Design review of the part built by this model. Coordinates are the model's own, in mm. A direction names the side the tool comes from. Coordinates: 2 decimals unless noted, no trailing zeros. Order: outer loops, then holes, each group sorted by start corner. A loop starts at its lowest first (then second) coordinate and runs counter-clockwise, first axis right, second up. Notation, with made-up numbers: (4.5, 70) -> (25.5, 70) arc R30 ccw to (25.5, 109) -> close; hole circle Ø1 at (10.5, 38). An arc over 180 degrees is marked (long way). Write item = value, one per line.
```python
from build123d import *

# Parameters (mm, degrees)
SKETCH_1_W      = 50
SKETCH_1_H      = 70
SKETCH_1_R      = 2.15
SKETCH_1_W_2    = 3.5
SKETCH_1_H_2    = 45
EXTRUDE_1_DEPTH = 5
FILLET_1_R      = 2
FILLET_2_R      = 2


with BuildPart() as part:
    # 草圖1 → 填料-伸長1 (new body)
    with BuildSketch(Plane(origin=(0, 0, 0), x_dir=(1, 0, 0), z_dir=(0, 1, 0))):
        Rectangle(SKETCH_1_W, SKETCH_1_H)
        with Locations(Location((-15.5, 25, 0), (0, 0, 270))):
            Circle(SKETCH_1_R, mode=Mode.SUBTRACT)
        with Locations(Location((15.5, 25, 0), (0, 0, 270))):
            Circle(SKETCH_1_R, mode=Mode.SUBTRACT)
        with Locations((-15.1, -7.5)):
            Rectangle(SKETCH_1_W_2, SKETCH_1_H_2, mode=Mode.SUBTRACT)
        with Locations((15.1, -7.5)):
            Rectangle(SKETCH_1_W_2, SKETCH_1_H_2, mode=Mode.SUBTRACT)
    extrude(amount=EXTRUDE_1_DEPTH)

    # 圓角1
    # the kernel refuses this fillet: 2 mm, written as the material it adds along each edge
    with BuildSketch(Plane(origin=(16.85, 0, 30), x_dir=(0, 0, -1), z_dir=(0, 1, 0)), Plane(origin=(-13.35, 0, 30), x_dir=(0, 0, -1), z_dir=(0, 1, 0))) as fillet_1_piece_1:
        with BuildLine():
            CenterArc((FILLET_1_R, FILLET_1_R), FILLET_1_R, 180, 90)
            Line((0, FILLET_1_R), (0, 0))
            Line((0, 0), (FILLET_1_R, 0))
        make_face()
    extrude(amount=5)
    with BuildSketch(Plane(origin=(13.35, 0, 30), x_dir=(0, 0, -1), z_dir=(0, 1, 0)), Plane(origin=(-16.85, 0, 30), x_dir=(0, 0, -1), z_dir=(0, 1, 0)), Plane(origin=(16.85, 0, -15), x_dir=(0, 0, 1), z_dir=(0, 1, 0)), Plane(origin=(13.35, 0, -15), x_dir=(1, 0, 0), z_dir=(0, 1, 0)), Plane(origin=(-13.35, 0, -15), x_dir=(0, 0, 1), z_dir=(0, 1, 0)), Plane(origin=(-16.85, 0, -15), x_dir=(1, 0, 0), z_dir=(0, 1, 0))) as fillet_1_piece_2:
        with BuildLine():
            CenterArc((FILLET_1_R, -FILLET_1_R), FILLET_1_R, 90, 90)
            Line((0, -FILLET_1_R), (0, 0))
            Line((0, 0), (FILLET_1_R, 0))
        make_face()
    extrude(amount=5)

    # 圓角2
    fillet_2_edges = [part.edges().sort_by_distance(p)[0] for p in [
        (25, 2.5, 35),
        (-25, 2.5, 35),
        (-25, 2.5, -35),
        (25, 2.5, -35),
    ]]
    fillet(fillet_2_edges, radius=FILLET_2_R)


solid = part.part
```
(1) We need section C-C (z = -25). Write out the cut boundary in (x, y).
Report:
outline = (-25, 0) -> (-17.65, 0) -> (-17.65, 5) -> (-25, 5) -> close; (-13.35, 0) -> (13.35, 0) -> (13.35, 5) -> (-13.35, 5) -> close; (17.65, 0) -> (25, 0) -> (25, 5) -> (17.65, 5) -> close
(2) We need section B-B (z = 8). Write out the cut boundary in (x, y), and give its area (3 significant figures).
Report:
outline = (-25, 0) -> (-16.85, 0) -> (-16.85, 5) -> (-25, 5) -> close; (-13.35, 0) -> (13.35, 0) -> (13.35, 5) -> (-13.35, 5) -> close; (16.85, 0) -> (25, 0) -> (25, 5) -> (16.85, 5) -> close
area = 215 mm²
(3) We need section A-A (y = 3.3). Write out the cut boundary in (x, z).
Report:
outline = (-25, -33) arc R2 ccw to (-23, -35) -> (23, -35) arc R2 ccw to (25, -33) -> (25, 33) arc R2 ccw to (23, 35) -> (-23, 35) arc R2 ccw to (-25, 33) -> close; hole circle Ø4.3 at (-15.5, -25); hole (-16.85, -13) arc R2 ccw to (-15.1, -14.98) arc R2 ccw to (-13.35, -13) -> (-13.35, 28) arc R2 ccw to (-15.1, 29.98) arc R2 ccw to (-16.85, 28) -> close; hole circle Ø4.3 at (15.5, -25); hole (13.35, -13) arc R2 ccw to (15.1, -14.98) arc R2 ccw to (16.85, -13) -> (16.85, 28) arc R2 ccw to (15.1, 29.98) arc R2 ccw to (13.35, 28) -> close
(4) For faces 1 (the flat face through (0, 5, 0)), 2 (the cylindrical face through (13.863, 2.465, -14.338)), list the 3-axis set-ups (+Z, -Z, +X, -X, +Y, -Y) from which the entire face can be reached by the end or side of a thin tool; tool diameter is ignored.
Report:
face_1 = +Z, -Z, +X, -X, +Y
face_2 = +Y, -Y
(5) For L1, parallel to X at y = 3.1, z = -25; L2, parallel to X at y = 4.8, z = 4; L3, parallel to Z at x = 14.5, y = 4.55, list the stretches that pass through material, from the lowest coordinate up.
Report:
L1 = -25 to -17.65, -13.35 to 13.35, 17.65 to 25
L2 = -25 to -16.85, -13.35 to 13.35, 16.85 to 25
L3 = -35 to -26.9, -23.1 to -14.81, 29.81 to 35
(6) The part is to be moulded in two halves that separate along X. For faces 3 (the cylindrical face through (24.4, 2.54, -34.43)), 4 (the cylindrical face through (-13.84, 2.46, -14.31)), 5 (the flat face through (0, 2, 35)), say which applies: released by +X, released by -X, zero draft, split by the parting line, or undercut.
Report:
face_3 = released by +X
face_4 = undercut
face_5 = zero draft
